The model under review builds one solid part; all positions refer to its coordinate system, in mm. A direction names the side the tool comes from. Round coordinates to 2 decimals unless told otherwise and drop trailing zeros. Order: outer loops, then holes, each group sorted by start corner. A loop starts at its lowest first (then second) coordinate and runs counter-clockwise, first axis right, second up.
Autodesk Inventor part; units mm, degrees
ref_plane "YZ Plane" through (0, 0, 0) normal (1, 0, 0) x (0, 1, 0)
ref_plane "XZ Plane" through (0, 0, 0) normal (0, 1, 0) x (-1, 0, 0)
ref_plane "XY Plane" through (0, 0, 0) normal (0, 0, 1) x (1, 0, 0)
sketch "Sketch1" plane through (0, 0, 0) normal (0, 0, 1) x (1, 0, 0)
  circle A0 centre (0, 0) radius 7
  circle A1 centre (0, 0) radius 2.3
  circle A2 centre (0, 0) radius 3.11
  dimension "d0" = 14
  dimension "d1" = 4.6
  dimension "d2" = 6.22
extrude "Extrusion1" add sketch "Sketch1" against normal blind 4.06 contours A0 | A1 | A2
extrude "Extrusion2" add sketch "Sketch1" along normal blind 9.82 contours A1 | A2
extrude "Extrusion3" cut sketch "Sketch1" along normal blind 4.82 contours A2
sketch "Sketch2" plane through (0, 0, -4.06) normal (0, 0, -1) x (-1, 0, 0)
  line L0 (7, 1) -> (-7, 1)
  line L1 (-7, 1) -> (-7, -1)
  line L2 (-7, -1) -> (7, -1)
  line L3 (7, -1) -> (7, 1)
  line L4 (7, 1) -> (-7, -1) construction
  line L5 (-7, 1) -> (7, -1) construction
  point P0 (0, 0)
  dimension "d9" = 2
extrude "Extrusion4" cut sketch "Sketch2" against normal blind 2
chamfer "Chamfer1" distance 1 angle 45 2 edges at (0, -7, -4.06) (0, 7, -4.06)
properties part number "AccessoryScrew"
(1) Draft analysis for pull direction Z (two halves, no side actions). For faces 1 (the cylindrical face through (-1.825, 1.4, 2.376)), 2 (the conical face through (0.12, 6.17, -3.89)), 3 (the flat face through (0, 0, 9.82)), state which applies: pulls with the +Z half, pulls with the -Z half, needs draft (parallel to the pull), parting line crosses it, or undercut.
Data:
face 1: undercut
face 2: pulls with the -Z half
face 3: pulls with the +Z half
(2) For faces 4 (the cylindrical face through (-0.674, 3.036, 7.285)), 5 (the flat face through (0, 3, -4.06)), 6 (the flat face through (0, 0, -2.06)), list the 3-axis set-ups (+Z, -Z, +X, -X, +Y, -Y) from which the entire face can be reached by the end or side of a thin tool; tool diameter is ignored.
Data:
face 4: +Z
face 5: -Z, +X, -X, +Y, -Y
face 6: -Z, +X, -X
(3) To check wall thickness, follow probe 1 along Z at (x, y) = (-0.5, 0); probe 2 along Z at (x, y) = (-4.5, -1.5); probe 3 along Y at (x, z) = (1.5, -2.25). State the ranges of each line that lie inside material, in increasing order.
Data:
probe 1: z = -2.06 to 9.82
probe 2: z = -4.06 to 0
probe 3: y = -6.84 to -1, 1 to 6.84
(4) Consider section C-C (z = 1.5). Write out the cut boundary in (x, y), and give its area (3 significant figures).
Data:
outline: circle Ø4.6 at (0, 0)
area: 16.6 mm2
(5) Consider section A-A (y = 0). Write out the cut boundary in (x, z), and give its area (3 significant figures).
Data:
outline: (-7, -2.06) - (7, -2.06) - (7, 0) - (2.3, 0) - (2.3, 4.82) - (3.11, 4.82) - (3.11, 9.82) - (-3.11, 9.82) - (-3.11, 4.82) - (-2.3, 4.82) - (-2.3, 0) - (-7, 0) - close
area: 82.1 mm2
(6) Insertion check: pin 1 (1 mm diameter, centred on x = 3, y = 0, fed in from -Z); pin 2 (3 mm diameter, centred on y = -5.5, z = -1, fed in from -X); pin 3 (1.6 mm diameter, centred on x = 2, z = -3.5, fed in from -Y). Each pin has a flat end and moves straight along its axis. Give the tip position at first contact, or say it passes through.
Data:
pin 1: stops at z = -2.06
pin 2: stops at x = -5.74
pin 3: stops at y = -6.87
(7) Consider section B-B (x = 0). Write out the cut boundary in (y, z), and give its area (3 significant figures).
Data:
outline: (-7, -3.06) - (-6, -4.06) - (-1, -4.06) - (-1, -2.06) - (1, -2.06) - (1, -4.06) - (6, -4.06) - (7, -3.06) - (7, 0) - (2.3, 0) - (2.3, 4.82) - (3.11, 4.82) - (3.11, 9.82) - (-3.11, 9.82) - (-3.11, 4.82) - (-2.3, 4.82) - (-2.3, 0) - (-7, 0) - close
area: 105 mm2
